Geometry: final body of the model. Coordinates: model frame, mm. Face numbers are marked on the shaded views. A direction names the side the tool comes from. Coordinates: 2 decimals unless noted, no trailing zeros. Loops run counter-clockwise (first coordinate to the right, second up) from the corner with the lowest first, then second, coordinate; pieces in that order, holes last. Notation, with made-up numbers: (46, -33) - (54, -33) arc R24 cw to (54, -18) - close; hole circle Ø5 at (34, 59.5). An arc over 180 degrees is marked (long way). Put each result on its own line as item: value. Start each with the question number.
1) Section D-D on x = -11.5. Output: boundary loops of the cut face in (y, z).
2) Contact query for flat-ended pins moving along their axis: pin 1 Ø3 at (x, z) = (2.5, 6.5) entering from +Y; pin 2 Ø9.5 at (x, z) = (-39.5, 12) entering from -Y; pin 3 Ø2 at (y, z) = (-33, 8) entering from +X. Output: stop coordinate, or through.
3) Draft query along Y for the marked faces 1, 2 and 3. Return one class per face: +Y half, -Y half, draft (parallel to the pull), parting line (faces both ways), or undercut.
4) Material intervals for line 1 along Y through (x, z) = (40.5, 15); line 2 along Y through (x, z) = (0, 14); line 3 along X through (y, z) = (39.5, 3.25), sorted ascending. Write a range as from..to.
5) Section A-A on y = 0. Output: boundary loops of the cut face in (x, z).
6) Reachability of the marked faces 4, 5, 6, 7 and 8 from +Z, -Z, +X, -X, +Y, -Y: full face, straight path, thin tool, end or side. Return the list, or none.
7) Section B-B on x = 0. Output: boundary loops of the cut face in (y, z).
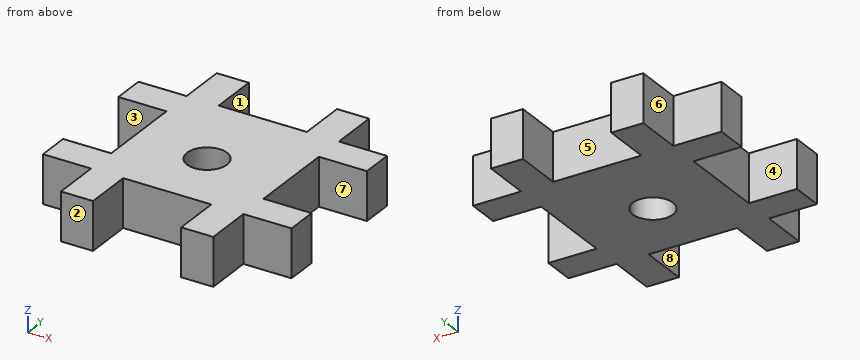
```python
from build123d import *

# Parameters (mm, degrees)
F0_W     = 98.425
F0_H     = 98.425
F1_DEPTH = 19.05
F2_W     = 19.05
F2_H     = 19.05
F2_H_2   = 34.925
F2_W_2   = 34.925
F3_DEPTH = 19.051
F4_R     = 7.9375
F5_DEPTH = 19.051


with BuildPart() as f1:
    # F0 (on Top) → F1 (new body)
    with BuildSketch(Plane.XY):
        with Locations((0.8939672261, 3.5788302732)):
            Rectangle(F0_W, F0_H)
    extrude(amount=F1_DEPTH)

    # F2 (on face) → F3 (cut, through all)
    with BuildSketch(Plane.XY.offset(19.05)):
        with Locations((-38.7935327739, 43.2663302732)):
            Rectangle(F2_W, F2_H)
        with Locations((40.5814672261, 43.2663302732)):
            Rectangle(F2_W, F2_H)
        with Locations((-38.7935327739, -36.1086697268)):
            Rectangle(F2_W, F2_H)
        with Locations((40.5814672261, -36.1086697268)):
            Rectangle(F2_W, F2_H)
        with Locations((40.5814672261, 3.5788302732)):
            Rectangle(F2_W, F2_H_2)
        with Locations((-38.7935327739, 3.5788302732)):
            Rectangle(F2_W, F2_H_2)
        with Locations((0.8939672261, 43.2663302732)):
            Rectangle(F2_W_2, F2_H)
        with Locations((0.8939672261, -36.1086697268)):
            Rectangle(F2_W_2, F2_H)
    extrude(amount=-F3_DEPTH, mode=Mode.SUBTRACT)

    # F4 (on face) → F5 (cut, through all)
    with BuildSketch(Plane.XY.offset(19.05)):
        Circle(F4_R)
    extrude(amount=-F5_DEPTH, mode=Mode.SUBTRACT)


solid = f1.part
```
Answer block:
1. outline: (-26.58, 0) - (33.74, 0) - (33.74, 19.05) - (-26.58, 19.05) - close
2. pin 1: stops at y = 33.74
2. pin 2: stops at y = -26.58
2. pin 3: stops at x = 31.06
3. face 1: draft
3. face 2: -Y half
3. face 3: undercut
4. line 1: y = -26.58..-13.88, 21.04..33.74
4. line 2: y = -26.58..-7.94, 7.94..33.74
4. line 3: x = -29.27..-16.57, 18.36..31.06
5. outline: (-29.27, 0) - (-7.94, 0) - (-7.94, 19.05) - (-29.27, 19.05) - close; (7.94, 0) - (31.06, 0) - (31.06, 19.05) - (7.94, 19.05) - close
6. face 4: +Z, -Z, -X
6. face 5: +Z, -Z, +Y
6. face 6: +Z, -Z, -X, +Y
6. face 7: +Z, -Z, +X
6. face 8: +Z, -Z, -Y
7. outline: (-26.58, 0) - (-7.94, 0) - (-7.94, 19.05) - (-26.58, 19.05) - close; (7.94, 0) - (33.74, 0) - (33.74, 19.05) - (7.94, 19.05) - close
